For this review, take the finished solid that the model builds, in its own axes (mm). A direction names the side the tool comes from. Round coordinates to 2 decimals unless told otherwise and drop trailing zeros. Loops run counter-clockwise (first coordinate to the right, second up) from the corner with the lowest first, then second, coordinate; pieces in that order, holes last.
1) Mouldability with a two-part tool opening along X and no side actions: class faces 3 (the flat face through (-10, 0, 40)), 4 (the cylindrical face through (-0.22, 0.07, 79.392)), 5 (the flat face through (0, -5, 40)), 6 (the cylindrical face through (-3.955, 2.535, 5.745)) as pulls with the +X half, pulls with the -X half, needs draft (parallel to the pull), parting line crosses it, or undercut.
2) Take a section at C-C (z = 70.5). State the section outline as (x, y) points, then the cut area to 3 significant figures.
3) Take a section at D-D (x = 3.5). State the section outline as (y, z) points.
4) Insertion check: pin 1 (1.5 mm diameter, centred on x = -2.5, z = 70.5, fed in from -Y); pin 2 (4 mm diameter, centred on x = 1.5, z = 8.5, fed in from +Y); pin 3 (1 mm diameter, centred on x = 4.5, y = -2, fed in from -Z); pin 4 (5 mm diameter, centred on x = -7, y = -1, fed in from +Z). Each pin has a flat end and moves straight along its axis. Give the tip position at first contact, or say it passes through.
5) Take a section at A-A (x = 0). State the section outline as (y, z) points.
6) Tool access review of faces 1 (the flat face through (10, 0, 40)), 2 (the flat face through (-1, 0, 6)): name each direction out of +Z, -Z, +X, -X, +Y, -Y from which nothing blocks a thin tool from reaching the whole face with its end or side.
7) Take a section at B-B (y = 1.5). State the section outline as (x, z) points, then the cut area to 3 significant figures.
8) Wall thickness on L1, parallel to Z at x = 1, y = 0.5; L2, parallel to Z at x = -2.5, y = 1; L3, parallel to X at y = 1.75, z = 11.5: over which ranges is each line inside the solid? List them lowest first.
```python
from build123d import *

# Parameters (mm, degrees)
SKETCH_1_W          = 20
SKETCH_1_H          = 10
EXTRUDE_1_DEPTH     = 80.297387422
SKETCH_2_R          = 6.5
CUT_EXTRUDE_1_DEPTH = 5
SKETCH_3_R          = 4.5
CUT_EXTRUDE_2_DEPTH = 20


with BuildPart() as part:
    # 스케치1 → 보스-돌출1 (new body)
    with BuildSketch(Plane.XY):
        Rectangle(SKETCH_1_W, SKETCH_1_H)
    extrude(amount=EXTRUDE_1_DEPTH)

    # 스케치2 → 컷-돌출1 (cut)
    with BuildSketch(Plane(origin=(0, 5, 0), x_dir=(1, 0, 0), z_dir=(0, 1, 0))):
        with Locations(Location((0, -10.902706153, 0), (0, 0, 270))):
            Circle(SKETCH_2_R)
    cut_extrude_1 = extrude(amount=-CUT_EXTRUDE_1_DEPTH, mode=Mode.SUBTRACT)

    # 스케치3 → 컷-돌출2 (cut)
    with BuildSketch(Plane(origin=(0, 5, 0), x_dir=(1, 0, 0), z_dir=(0, 1, 0))):
        with Locations(Location((0, -10.902706153, 0), (0, 0, 270))):
            Circle(SKETCH_3_R)
        with BuildLine():
            Line((-21.262122506, -10.902706153), (-10, -10.902706153))
            ThreePointArc((-10, -10.902706153), (0, -0.902706153), (10, -10.902706153))
            Line((10, -10.902706153), (21.262122506, -10.902706153))
            ThreePointArc((21.262122506, -10.902706153), (0, 10.359416353), (-21.262122506, -10.902706153))
        make_face()
    cut_extrude_2 = extrude(amount=-CUT_EXTRUDE_2_DEPTH, mode=Mode.SUBTRACT)

    # 대칭 복사1: 컷-돌출1, 컷-돌출2 across plane
    add(cut_extrude_1.mirror(Plane.XY.offset(40.148693711)), mode=Mode.SUBTRACT)
    add(cut_extrude_2.mirror(Plane.XY.offset(40.148693711)), mode=Mode.SUBTRACT)


solid = part.part
```
Response:
1. face 3: pulls with the -X half
1. face 4: parting line crosses it
1. face 5: needs draft
1. face 6: undercut
2. outline: (-9.94, -5) - (-4.36, -5) - (-4.36, 0) - (-6.41, 0) - (-6.41, 5) - (-9.94, 5) - close; (4.36, -5) - (9.94, -5) - (9.94, 5) - (6.41, 5) - (6.41, 0) - (4.36, 0) - close
2. area: 91.1 mm2
3. outline: (-5, 1.54) - (5, 1.54) - (5, 5.43) - (0, 5.43) - (0, 8.07) - (-5, 8.07) - close; (-5, 13.73) - (0, 13.73) - (0, 16.38) - (5, 16.38) - (5, 63.92) - (0, 63.92) - (0, 66.57) - (-5, 66.57) - close; (-5, 72.22) - (0, 72.22) - (0, 74.87) - (5, 74.87) - (5, 78.76) - (-5, 78.76) - close
4. pin 1: passes through
4. pin 2: stops at y = 0
4. pin 3: stops at z = 1.74
4. pin 4: stops at z = 78.32
5. outline: (-5, 0.9) - (5, 0.9) - (5, 4.4) - (0, 4.4) - (0, 6.4) - (-5, 6.4) - close; (-5, 15.4) - (0, 15.4) - (0, 17.4) - (5, 17.4) - (5, 62.89) - (0, 62.89) - (0, 64.89) - (-5, 64.89) - close; (-5, 73.89) - (0, 73.89) - (0, 75.89) - (5, 75.89) - (5, 79.39) - (-5, 79.39) - close
6. face 1: +Z, -Z, +X, +Y, -Y
6. face 2: +Y
7. outline: (-10, 10.9) arc R10 ccw to (10, 10.9) - (10, 69.39) arc R10 ccw to (-10, 69.39) - close; hole circle Ø13 at (0, 10.9); hole circle Ø13 at (0, 69.39)
7. area: 1,220 mm2
8. L1: z = 0.95 to 4.48, 17.33 to 62.97, 75.82 to 79.34
8. L2: z = 1.22 to 4.9, 16.9 to 63.39, 75.39 to 79.08
8. L3: x = -10 to -6.47, 6.47 to 10
